Source: three-view drawing plus pictorial views. Frame: mm from the lowest corner of the part. A direction names the side the tool comes from. Coordinates: 2 decimals unless noted, no trailing zeros. Order: outer loops, then holes, each group sorted by start corner. A loop starts at its lowest first (then second) coordinate and runs counter-clockwise, first axis right, second up. Notation, with made-up numbers: (-8.5, 37.25) -> (-2.5, 37.25) arc R24 ccw to (-2.5, 54.25) -> close; hole circle Ø1 at (28, -13). An arc over 180 degrees is marked (long way). Use one line per item in the form item = value. Start each with the question number.
1) Section query A-A on x = 36. Count the separate pieces of the cut face and the enclosed holes in it, then the cut area to 3 significant figures.
2) Access query for the marked faces 1, 2 and 3. Directions: +Z, -Z, +X, -X, +Y, -Y. A direction counts if a zero-diameter tool reaches every point of the face in a straight line with its end or side. Return the directions, or none.
3) Section query D-D on y = 27. Output: boundary loops of the cut face in (x, z).
4) Pin query (flat end, axial travel): pin 1 (4 mm diameter, centred on x = 55.5, y = 31, fed in from +Z); pin 2 (5 mm diameter, centred on x = 15.5, z = 27, fed in from -Y); pin 3 (10 mm diameter, centred on x = 48, z = 32.5, fed in from +Y). Return the tip coordinate at first contact, or that it passes through.
5) Section query B-B on z = 36. Output: boundary loops of the cut face in (x, y).
6) Draft query along Z for the marked faces 4, 5, 6 and 7. Return one class per face: pulls with the +Z half, pulls with the -Z half, needs draft (parallel to the pull), parting line crosses it, or undercut.
7) Section query C-C on z = 7.5. Output: boundary loops of the cut face in (x, y), then the cut area to 3 significant figures.
8) Ray query, line 1 along Y through (x, z) = (61, 13); line 2 along X through (y, z) = (27, 50) (1 decimal); line 3 along Y through (x, z) = (20.5, 25). Return the intervals inside material, ascending.
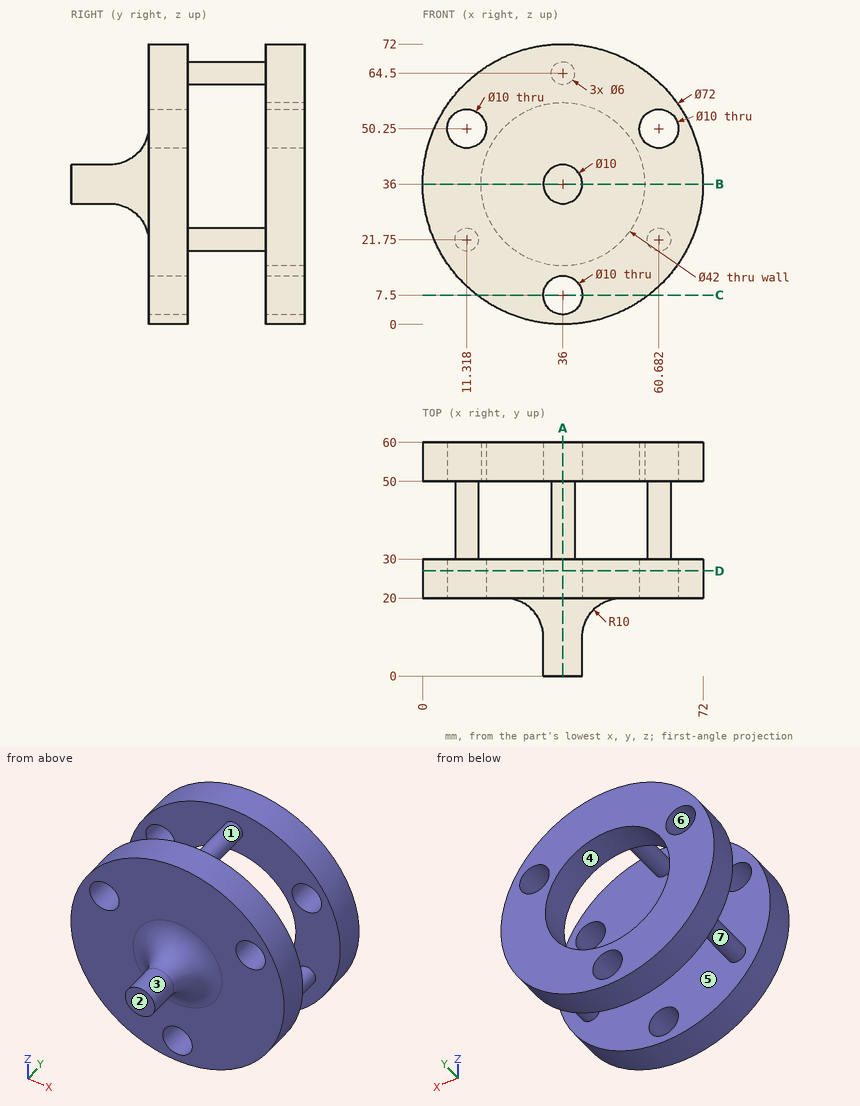
Answers below:
q1.separate_pieces = 4
q1.enclosed_holes = 0
q1.area = 1,180 mm^2
q2.face_1 = none
q2.face_2 = +Z, -Z, +X, -X, -Y
q2.face_3 = -Y
q3.outline = circle Ø72 at (36, 36); hole circle Ø10 at (11.32, 50.25); hole circle Ø10 at (36, 7.5); hole circle Ø10 at (60.68, 50.25)
q4.pin_1 = 67.31
q4.pin_2 = 20
q4.pin_3 = 30
q5.outline = (0, 20) -> (21, 20) arc R10 cw to (31, 10) -> (31, 0) -> (41, 0) -> (41, 10) arc R10 cw to (51, 20) -> (72, 20) -> (72, 30) -> (0, 30) -> close; (0, 50) -> (15, 50) -> (15, 60) -> (0, 60) -> close; (57, 50) -> (72, 50) -> (72, 60) -> (57, 60) -> close
q6.face_4 = undercut
q6.face_5 = needs draft
q6.face_6 = undercut
q6.face_7 = parting line crosses it
q7.outline = (14.01, 20) -> (31, 20) -> (31, 30) -> (14.01, 30) -> close; (14.01, 50) -> (31, 50) -> (31, 60) -> (14.01, 60) -> close; (41, 20) -> (57.99, 20) -> (57.99, 30) -> (41, 30) -> close; (41, 50) -> (57.99, 50) -> (57.99, 60) -> (41, 60) -> close
q7.area = 680 mm^2
q8.line_1 = 20 to 30, 50 to 60
q8.line_2 = 2.8 to 6.3, 16.3 to 55.7, 65.7 to 69.2
q8.line_3 = 20 to 30
